Design review of the part built by this model. Coordinates are the model's own, in mm. Face numbers are marked on the shaded views. A direction names the side the tool comes from. Coordinates: 2 decimals unless noted, no trailing zeros. Loops run counter-clockwise (first coordinate to the right, second up) from the corner with the lowest first, then second, coordinate; pieces in that order, holes last. Notation, with made-up numbers: M -5,-36.5 L 39,-36.5 A31 cw 39,-8.5 Z; hole C 71.25,43.25 d7. An arc over 180 degrees is marked long. Write item = value, one per line. Start each with the question number.
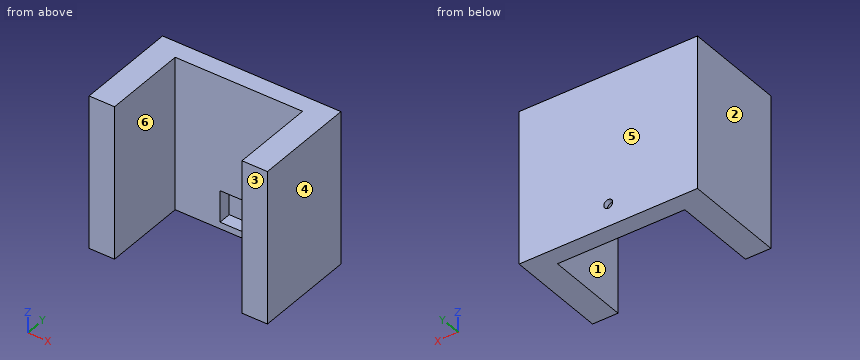
from build123d import *

# Parameters (mm, degrees)
BOSS_EXTRUDE1_DEPTH     = 60
CUT_EXTRUDE1_DEPTH      = 91.461766578
CUT_EXTRUDE1_DEPTH_BACK = 91.461766578
SKETCH2_R               = 1.75
SKETCH3_W               = 14.779269325
SKETCH3_H               = 12.394379378
CUT_EXTRUDE2_DEPTH      = 5


with BuildPart() as part:
    # Sketch1 → Boss-Extrude1 (new body)
    with BuildSketch(Plane.XY):
        Polygon((-59.112868416, -8.322842348), (-59.112868416, -48.322842348), (-49.112868416, -48.322842348), (-49.112868416, -15.322842348), (0.887131584, -15.322842348), (0.887131584, -48.322842348), (10.887131584, -48.322842348), (10.887131584, -8.322842348), align=None)
    extrude(amount=BOSS_EXTRUDE1_DEPTH)

    # Sketch2 → Cut-Extrude1 (cut, two sides: drawn at the far end of the back side and taken through both)
    with BuildSketch(Plane(origin=(0, -15.322842348, 0), x_dir=(1, 0, 0), z_dir=(0, 1, 0)).offset(-CUT_EXTRUDE1_DEPTH_BACK)):
        with Locations(Location((-24.112868416, -8.79280196, 0), (0, 0, 270))):
            Circle(SKETCH2_R)
    extrude(amount=CUT_EXTRUDE1_DEPTH + CUT_EXTRUDE1_DEPTH_BACK, mode=Mode.SUBTRACT)

    # Sketch3 → Cut-Extrude2 (cut)
    with BuildSketch(Plane(origin=(0, -15.322842348, 0), x_dir=(-1, 0, 0), z_dir=(0, -1, 0))):
        with Locations((24.112868416, -8.79280196)):
            Rectangle(SKETCH3_W, SKETCH3_H)
    extrude(amount=-CUT_EXTRUDE2_DEPTH, mode=Mode.SUBTRACT)


solid = part.part
Q1. Clearance check with flat-ended pins moving along their axes: P1, Ø12, axis at x = -22, z = 21, coming from the -Y side; P2, Ø10, axis at x = -2.5, y = -31, coming from the +Z side; P3, Ø3, axis at x = -24.11, z = 8.79, coming from the -Y side; P4, Ø10, axis at x = -23.5, z = 8, coming from the -Y side. State where each tip first meets the part, or that it passes through.
Q2. Add section C-C on z = 29. State the section outline as (x, y) points, plus the area to 3 significant figures.
Q3. Add section A-A on y = -14.5. State the section outline as (x, z) points.
Q4. Add section B-B on y = -42. State the section outline as (x, z) points.
Q5. For the marked faces 5 and 6, list the 3-axis set-ups (+Z, -Z, +X, -X, +Y, -Y) from which the entire face can be reached by the end or side of a thin tool; tool diameter is ignored.
Q6. Mouldability with a two-part tool opening along X and no side actions: class the marked faces 1, 2, 3 and 4 as released by +X, released by -X, zero draft, split by the parting line, or undercut.
Q7. Add section D-D on x = -21. State the section outline as (y, z) points, plus the area to 3 significant figures.
Q8. To check wall thickness, follow line 1 (X direction, y = -29, z = 9); line 2 (Y direction, x = -8.5, z = 27.5). State the ranges of each line that lie inside material, in increasing order. Write a range as from..to.
Values follow:
q1.P1 = -15.32
q1.P2 = 60
q1.P3 = through
q1.P4 = -10.32
q2.outline = M -59.11,-48.32 L -49.11,-48.32 L -49.11,-15.32 L 0.89,-15.32 L 0.89,-48.32 L 10.89,-48.32 L 10.89,-8.32 L -59.11,-8.32 Z
q2.area = 1,150 mm2
q3.outline = M -59.11,0 L 10.89,0 L 10.89,60 L -59.11,60 Z; hole M -31.5,2.6 L -16.72,2.6 L -16.72,14.99 L -31.5,14.99 Z
q4.outline = M -59.11,0 L -49.11,0 L -49.11,60 L -59.11,60 Z; M 0.89,0 L 10.89,0 L 10.89,60 L 0.89,60 Z
q5.face_5 = +Z, -Z, +X, -X, +Y
q5.face_6 = +Z, -Z, -Y
q6.face_1 = undercut
q6.face_2 = released by -X
q6.face_3 = zero draft
q6.face_4 = released by +X
q7.outline = M -15.32,0 L -8.32,0 L -8.32,60 L -15.32,60 L -15.32,14.99 L -10.32,14.99 L -10.32,2.6 L -15.32,2.6 Z
q7.area = 358 mm2
q8.line_1 = -59.11..-49.11, 0.89..10.89
q8.line_2 = -15.32..-8.32
